from build123d import *

# Parameters (mm, degrees)
F0_W     = 60
F0_H     = 80
F1_DEPTH = 20
F2_T     = -2.5
F3_W     = 11
F3_H     = 9
F4_DEPTH = 10
F5_W     = 2
F5_H     = 8
F6_DEPTH = 25
F7_R     = 2
F8_R     = 2


with BuildPart() as f1:
    # F0 (on Top) → F1 (new body)
    with BuildSketch(Plane.XY):
        with Locations((1.363532, 17.233828)):
            Rectangle(F0_W, F0_H)
    extrude(amount=F1_DEPTH)

    # F2
    f2_openings = [f1.faces().sort_by_distance(p)[0] for p in [
        (1.363532, 17.233828, 20),
    ]]
    offset(amount=F2_T, openings=f2_openings)

    # F3 (on face) → F4 (cut)
    with BuildSketch(Plane.XZ.offset(22.766172)):
        with Locations((-12.330356, 10.031623)):
            Rectangle(F3_W, F3_H)
    extrude(amount=-F4_DEPTH, mode=Mode.SUBTRACT)

    # F5 (on face) → F6 (cut)
    with BuildSketch(Plane(origin=(0, 57.233828, 0), x_dir=(-1, 0, 0), z_dir=(0, 1, 0))):
        with Locations((19.115507, 16)):
            Rectangle(F5_W, F5_H)
    extrude(amount=-F6_DEPTH, mode=Mode.SUBTRACT)

    # F7
    f7_edges = [f1.edges().sort_by_distance(p)[0] for p in [
        (31.363532, -22.766172, 10),
        (31.363532, 57.233828, 10),
        (-28.636468, 57.233828, 10),
        (-28.636468, -22.766172, 10),
    ]]
    fillet(f7_edges, radius=F7_R)

    # F8
    f8_edges = [f1.edges().sort_by_distance(p)[0] for p in [
        (1.363532, 57.233828, 0),
        (30.777745, 56.648042, 0),
        (-28.050682, 56.648042, 0),
        (31.363532, 17.233828, 0),
        (-28.636468, 17.233828, 0),
        (30.777745, -22.180386, 0),
        (-28.050682, -22.180386, 0),
        (1.363532, -22.766172, 0),
    ]]
    fillet(f8_edges, radius=F8_R)


solid = f1.part
Here's how the part is built. I have some questions about the finished solid (model axes, mm). A direction names the side the tool comes from. Give positions to 0.01 mm unless a question says otherwise; leave off trailing zeros. Loops run counter-clockwise (first coordinate to the right, second up) from the corner with the lowest first, then second, coordinate; pieces in that order, holes last. Notation, with made-up numbers: (15.25, 58.5) -> (26.25, 58.5) arc R22 cw to (26.25, 65.5) -> close; hole circle Ø4 at (22.5, 60). An arc over 180 degrees is marked (long way). Answer as a JSON object with one key per item and string values. Group by question number.
Item 1: Imagine slicing it at C-C on y = -14. Write out the boundary of the cut face in (x, z), then the cut area to 3 significant figures.
Item 2: On a 3-axis mill with a long thin cutter (end or side, diameter ignored), from which of +Z, -Z, +X, -X, +Y, -Y can I reach the whole of each face in a straight line? I mean faces 4 (the flat face through (1, 54.734, 11)), 5 (the flat face through (-20.116, 56, 16)), 6 (the flat face through (-6.83, -22, 10)). Say none if no direction works.
Item 3: Thinking about a two-plate mould opening in Y: for faces 1 (the flat face through (31.364, 17, 11)), 2 (the cylindrical face through (30.762, 56.664, 11.126)), 3 (the flat face through (28.864, 17, 11)), which applies, pulls with the +Y half, pulls with the -Y half, needs draft (parallel to the pull), parting line crosses it, or undercut?
Item 4: Imagine slicing it at B-B on z = 8.75. Write out the boundary of the cut face in (x, y).
Item 5: Imagine slicing it at A-A on x = -10.5. Write out the boundary of the cut face in (y, z).
Item 6: Imagine slicing it at D-D on x = -23. Write out the boundary of the cut face in (y, z), then the cut area to 3 significant figures.
Item 7: Will these pins go through, and if not, where does the flat tip stop? pin 1 (0.8 mm diameter, centred on y = -21.5, z = 9, fed in from -X); pin 2 (2 mm diameter, centred on y = -22, z = 10, fed in from +X); pin 3 (1.2 mm diameter, centred on x = -10, y = -21.5, fed in from -Z).
Item 8: I need wall thicknesses on L1, parallel to Y at x = 11.5, z = 8.5; L2, parallel to X at y = 53.5, z = 8.5; L3, parallel to Y at x = -20, z = 16.5. Which ranges of each line are inside material? Lowest first, please.
Answer list:
{
 "1": {"outline": "(-28.64, 2) arc R2 ccw to (-26.64, 0) -> (29.36, 0) arc R2 ccw to (31.36, 2) -> (31.36, 20) -> (28.86, 20) -> (28.86, 2.5) -> (-26.14, 2.5) -> (-26.14, 20) -> (-28.64, 20) -> close", "area": "236 mm2"},
 "2": {"face 4": "+Z", "face 5": "+Z, +Y", "face 6": "-Y"},
 "3": {"face 1": "needs draft", "face 2": "pulls with the +Y half", "face 3": "undercut"},
 "4": {"outline": "(-28.64, -20.77) arc R2 ccw to (-26.64, -22.77) -> (-17.83, -22.77) -> (-17.83, -20.27) -> (-26.14, -20.27) -> (-26.14, 54.73) -> (28.86, 54.73) -> (28.86, -20.27) -> (-6.83, -20.27) -> (-6.83, -22.77) -> (29.36, -22.77) arc R2 ccw to (31.36, -20.77) -> (31.36, 55.23) arc R2 ccw to (29.36, 57.23) -> (-26.64, 57.23) arc R2 ccw to (-28.64, 55.23) -> close"},
 "5": {"outline": "(-22.77, 2) arc R2 ccw to (-20.77, 0) -> (55.23, 0) arc R2 ccw to (57.23, 2) -> (57.23, 20) -> (54.73, 20) -> (54.73, 2.5) -> (-20.27, 2.5) -> (-20.27, 5.53) -> (-22.77, 5.53) -> close; (-22.77, 14.53) -> (-20.27, 14.53) -> (-20.27, 20) -> (-22.77, 20) -> close"},
 "6": {"outline": "(-22.77, 2) arc R2 ccw to (-20.77, 0) -> (55.23, 0) arc R2 ccw to (57.23, 2) -> (57.23, 20) -> (54.73, 20) -> (54.73, 2.5) -> (-20.27, 2.5) -> (-20.27, 20) -> (-22.77, 20) -> close", "area": "286 mm2"},
 "7": {"pin 1": "stops at x = -28.61", "pin 2": "stops at x = 31.35", "pin 3": "stops at z = 0"},
 "8": {"L1": "y = -22.77 to -20.27, 54.73 to 57.23", "L2": "x = -28.64 to -26.14, 28.86 to 31.36", "L3": "y = -22.77 to -20.27"}
}
